Autodesk Inventor part; units mm, degrees
ref_plane "YZ Plane" through (0, 0, 0) normal (1, 0, 0) x (0, 1, 0)
ref_plane "XZ Plane" through (0, 0, 0) normal (0, 1, 0) x (-1, 0, 0)
ref_plane "XY Plane" through (0, 0, 0) normal (0, 0, 1) x (1, 0, 0)
sketch "Sketch1" plane through (0, 0, 0) normal (0, 0, 1) x (1, 0, 0)
  line L0 (-4.5, -0.0453) -> (4.5, -0.0453)
  line L1 (4.5, -0.0453) -> (4.5, 0.8547)
  line L2 (4.5, 0.8547) -> (4.6, 0.8547)
  line L3 (6.5696, 2.5074) -> (10.5639, 25.1601)
  arc A0 (4.6, 0.8547) -> (6.5696, 2.5074) centre (4.6, 2.8547) ccw
  line L4 (-4.5, -0.0453) -> (-4.5, 0.8547)
  line L5 (-4.5, 0.8547) -> (-7.5, 0.8547)
  line L6 (-9.4696, 2.5074) -> (-13.4639, 25.1601)
  arc A1 (-9.4696, 2.5074) -> (-7.5, 0.8547) centre (-7.5, 2.8547) ccw
  line L7 (10.9778, 27.5074) -> (-13.8778, 27.5074) construction
  line L8 (-4.5, -0.7454) -> (-4.5, 29.497) construction
  line L9 (-4.5, 31.0971) -> (4.5, 31.0971) construction
  line L10 (4.5, 31.0971) -> (4.5, 0.8547) construction
  line L11 (8.5943, 27.5074) -> (4.5, 27.5074)
  line L12 (-11.4943, 27.5074) -> (-4.5, 27.5074)
  line L13 (4.5, 27.5074) -> (4.5, 28.4074)
  line L14 (-4.5, 28.4074) -> (-4.5, 27.5074)
  line L15 (-4.5, 28.4074) -> (4.5, 28.4074)
  arc A2 (10.5639, 25.1601) -> (8.5943, 27.5074) centre (8.5943, 25.5074) ccw
  arc A3 (-11.4943, 27.5074) -> (-13.4639, 25.1601) centre (-11.4943, 25.5074) ccw
  arc A4 (-3.3267, 6.6293) -> (-3.3267, 22.2828) centre (-3.3267, 14.456) ccw
  line L16 (-3.3267, 24.456) -> (-3.3267, 14.456)
  line L17 (-3.3267, 14.456) -> (-3.3267, 4.456)
  line L18 (-3.3267, 4.456) -> (-4.5, 4.456)
  line L19 (-3.3267, 24.456) -> (-4.5, 24.456)
  line L20 (-4.5, 4.4448) -> (-4.5, 24.4448)
  circle A5 centre (7.1554, 22.5114) radius 0.4516
  circle A6 centre (-1.2395, 24.4257) radius 0.9502
  circle A7 centre (-4.5, 27.0227) radius 0.3751
  point P0 (0, 0)
  dimension "d1" = 2
  dimension "d2" = 100
  dimension "d3" = 25
  dimension "d4" = 0.1
  dimension "d5" = 2
  dimension "d6" = 3
  dimension "d7" = 4.5
  dimension "d8" = 4.5
  dimension "d9" = 100
  dimension "d10" = 25
  dimension "d11" = 0.9
  dimension "d12" = 0.9
  dimension "d13" = 2
  dimension "d16" = 10
  dimension "d17" = 10
extrude "Extrusion1" add sketch "Sketch1" along normal mid plane 2 contours L4 L5 A1 L6 A3 L12 L14 L15 L13 L11 A2 L3 A0 L2 L1 L0 | L17 L16 A4 | A5 | A6 | A7
extrude "Extrusion2" cut sketch "Sketch1" against normal through all contours L17 L16 A4
extrude "Extrusion3" cut sketch "Sketch1" along normal through all both and the other way through all contours L17 L16 A4
extrude "Extrusion6" cut sketch "Sketch1" against normal through all both and the other way through all contours A6
extrude "Extrusion7" cut sketch "Sketch1" against normal through all both and the other way through all contours A7
sketch "Esboço2" plane through (4.5, -0.0453, 1) normal (1, 0, 0) x (0, 0, -1)
  line L0 (0, 0.9) -> (2, 0.9)
  line L1 (0, 0.9) -> (2, 0.9)
  line L2 (2, 0) -> (0, 0)
  line L3 (2, 0.9) -> (2, 0)
  line L4 (2, 0) -> (0, 0)
  line L5 (0, 0) -> (0, 0.9)
  line L6 (0, 0) -> (0, 0.9)
  point P0 (1, 0.0453)
extrude "Extrusão8" cut sketch "Esboço2" against normal blind 2
sketch "Esboço3" plane through (4.5, 27.5074, 1) normal (1, 0, 0) x (0, 0, -1)
  line L0 (2, 0.9) -> (0, 0.9)
  line L1 (0, 0.9) -> (2, 0.9)
  line L2 (2, 0) -> (0, 0)
  line L3 (2, 0.9) -> (2, 0)
  line L4 (2, 0) -> (0, 0)
  line L5 (0, 0.9) -> (0, 0)
  line L6 (0, 0) -> (0, 0.9)
  point P0 (1, -27.5074)
extrude "Extrusão9" cut sketch "Esboço3" against normal blind 1.5
sketch "Esboço4" plane through (0, 0, 1) normal (0, 0, 1) x (1, 0, 0)
  line L0 (-3.3267, 22.2828) -> (-3.3267, 6.6293)
  line L1 (-3.3267, 22.2828) -> (-3.3267, 24.456)
  line L2 (-3.3267, 24.456) -> (-4.8267, 24.456)
  line L3 (-4.8267, 24.456) -> (-4.8267, 4.456)
  line L4 (-4.8267, 4.456) -> (-3.3267, 4.456)
  line L5 (-3.3267, 4.456) -> (-3.3267, 6.6293)
  arc A0 (-3.3267, 6.6293) -> (-3.3267, 22.2828) centre (-3.3267, 14.456) ccw
  point P0 (0, 0)
  dimension "d36" = 20
  dimension "d37" = 1.5
  dimension "d38" = 10
extrude "Extrusão10" cut sketch "Esboço4" against normal blind 10 contours L0 L5 L4 L3 L2 L1
properties material "Liga de Nickel-Copper 400"
The listing builds one solid part. Answer for the finished solid, in the listing's coordinates (mm). A direction names the side the tool comes from. Coordinates: 2 decimals unless noted, no trailing zeros. Loops run counter-clockwise (first coordinate to the right, second up) from the corner with the lowest first, then second, coordinate; pieces in that order, holes last. Notation, with made-up numbers: (68, 30.25) - (95, 30.25) arc R30 ccw to (95, 52.25) - close; hole circle Ø5 at (62.25, 26.25). An arc over 180 degrees is marked (long way). Write item = value, one per line.
1) Find the intervals of material crossed by line 1 along Y through (x, z) = (-3.75, -0.4); line 2 along Y through (x, z) = (-1, -0.8); line 3 along Y through (x, z) = (-6.5, -0.25), in increasing order.
Responses:
line_1 = -0.05 to 4.46, 24.46 to 28.41
line_2 = -0.05 to 6.98, 21.93 to 23.51, 25.35 to 28.41
line_3 = 0.85 to 27.51
2) Which of the six approach directions +Z, -Z, +X, -X, +Y, -Y give full straight-line access (tool end or side, diameter ignored) to faces 4 (the face through (-6, 0.855, 0)), 5 (the face through (6, 27.507, 0)), 6 (the face through (4.5, 14.3, 0))?
Responses:
face_4 = +Z, -Z, -X, -Y
face_5 = +Z, -Z, +X, +Y
face_6 = +Z, -Z
3) Each of these flat-tipped pins is pushed along its axis until it touches: P1, Ø1, axis at x = -6.5, z = 0.5, coming from the -Y side; P2, Ø0.6, axis at y = 6, z = 0, coming from the -X side; P3, Ø1, axis at x = -7, z = -0.5, coming from the +Y side; P4, Ø1, axis at x = -4, y = 12.5, coming from the -Z side. Where does it stop, or does it pass through?
Responses:
P1 = 0.85
P2 = -10.14
P3 = 27.51
P4 = through
4) Section A-A (y = 19.5) is taken. Determine the outline of the cut face in (x, z).
Responses:
outline = (-12.47, -1) - (-4.83, -1) - (-4.83, 1) - (-12.47, 1) - close; (2.66, -1) - (9.57, -1) - (9.57, 1) - (2.66, 1) - close
5) Determine the mould class of faces 1 (the face through (-4.5, 28, 0)), 2 (the face through (-4.827, 15, 0)), 3 (the face through (-8, 27.507, 0)) for opening direction X: pulls with the +X half, pulls with the -X half, needs draft (parallel to the pull), parting line crosses it, or undercut.
Responses:
face_1 = pulls with the -X half
face_2 = undercut
face_3 = needs draft
6) Section C-C (y = 8.5) is taken. Determine the outline of the cut face in (x, z), plus the area to 3 significant figures.
Responses:
outline = (-10.53, -1) - (-4.83, -1) - (-4.83, 1) - (-10.53, 1) - close; (1.75, -1) - (7.63, -1) - (7.63, 1) - (1.75, 1) - close
area = 23.1 mm^2
7) Section D-D (y = 3) is taken. Determine the outline of the cut face in (x, z), plus the area to 3 significant figures.
Responses:
outline = (-9.56, -1) - (6.66, -1) - (6.66, 1) - (-9.56, 1) - close
area = 32.4 mm^2
